from build123d import *

# Parameters (mm, degrees)
SKETCH1_R           = 5.5
BOSS_EXTRUDE1_DEPTH = 14
SKETCH2_R           = 5.5
BOSS_EXTRUDE2_DEPTH = 13.52
SKETCH3_R           = 5.5
BOSS_EXTRUDE3_DEPTH = 5.8
SKETCH4_R           = 1.05
CUT_EXTRUDE1_DEPTH  = 3.5


with BuildPart() as part:
    # Sketch1 → Boss-Extrude1 (new body)
    with BuildSketch(Plane.YZ):
        with Locations(Location((0, 0, 0), (0, 0, 270))):
            Circle(SKETCH1_R)
        with BuildLine():
            Line((-1.747140521, 2.5), (1.747140521, 2.5))
            ThreePointArc((1.747140521, 2.5), (0, -3.05), (-1.747140521, 2.5))
        make_face(mode=Mode.SUBTRACT)
    extrude(amount=BOSS_EXTRUDE1_DEPTH)

    # Sketch2 → Boss-Extrude2 (add)
    with BuildSketch(Plane.YZ.offset(14)):
        with Locations(Location((0, 0, 0), (0, 0, 270))):
            Circle(SKETCH2_R)
    extrude(amount=BOSS_EXTRUDE2_DEPTH)

    # Sketch3 → Boss-Extrude3 (add)
    with BuildSketch(Plane.YZ.offset(27.52)):
        with Locations(Location((0, 0, 0), (0, 0, 270))):
            Circle(SKETCH3_R)
        with BuildLine():
            ThreePointArc((-1.322019746, -2.893008891), (-1.318956528, -2.868853063), (-1.317084788, -2.844575833))
            ThreePointArc((-1.317084788, -2.844575833), (-1.543809469, -2.402214423), (-2.040380396, -2.37974197))
            ThreePointArc((-2.040380396, -2.37974197), (-2.061686193, -2.391529691), (-2.0823866, -2.404350785))
            ThreePointArc((-2.0823866, -2.404350785), (-2.380259348, -2.555545236), (-2.703854763, -2.638454478))
            ThreePointArc((-2.703854763, -2.638454478), (-2.855120731, -2.473976197), (-2.996397469, -2.300842198))
            ThreePointArc((-2.996397469, -2.300842198), (-2.868279694, -1.992339732), (-2.676232473, -1.719016114))
            ThreePointArc((-2.676232473, -1.719016114), (-2.660595904, -1.700351039), (-2.645896034, -1.680939672))
            ThreePointArc((-2.645896034, -1.680939672), (-2.597470339, -1.186224957), (-3.003062861, -0.898853414))
            ThreePointArc((-3.003062861, -0.898853414), (-3.02735936, -0.897251093), (-3.051705258, -0.896845399))
            ThreePointArc((-3.051705258, -0.896845399), (-3.384033651, -0.862996099), (-3.701083558, -0.757794901))
            ThreePointArc((-3.701083558, -0.757794901), (-3.739412915, -0.537646409), (-3.764659163, -0.315616851))
            ThreePointArc((-3.764659163, -0.315616851), (-3.490090608, -0.12535376), (-3.1807603, 0.000752133))
            ThreePointArc((-3.1807603, 0.000752133), (-3.157514879, 0.008000426), (-3.134653985, 0.016382957))
            ThreePointArc((-3.134653985, 0.016382957), (-2.82645273, 0.406382552), (-3.012294086, 0.86741475))
            ThreePointArc((-3.012294086, 0.86741475), (-3.031867321, 0.881898388), (-3.052129059, 0.895402065))
            ThreePointArc((-3.052129059, 0.895402065), (-3.31340118, 1.103548202), (-3.523244473, 1.363459202))
            ThreePointArc((-3.523244473, 1.363459202), (-3.43646792, 1.569382314), (-3.337668173, 1.769814617))
            ThreePointArc((-3.337668173, 1.769814617), (-3.003822413, 1.781431146), (-2.675419206, 1.720281583))
            ThreePointArc((-2.675419206, 1.720281583), (-2.65194519, 1.713811812), (-2.628181444, 1.708504114))
            ThreePointArc((-2.628181444, 1.708504114), (-2.158056349, 1.869966471), (-2.065143222, 2.35828486))
            ThreePointArc((-2.065143222, 2.35828486), (-2.07377883, 2.381051361), (-2.083523449, 2.4033657))
            ThreePointArc((-2.083523449, 2.4033657), (-2.190787246, 2.719723746), (-2.226800162, 3.051824643))
            ThreePointArc((-2.226800162, 3.051824643), (-2.042468641, 3.178143241), (-1.850991121, 3.293342448))
            ThreePointArc((-1.850991121, 3.293342448), (-1.563861826, 3.12262425), (-1.320651417, 2.893633786))
            ThreePointArc((-1.320651417, 2.893633786), (-1.304401641, 2.875500057), (-1.287279864, 2.858187286))
            ThreePointArc((-1.287279864, 2.858187286), (-0.804492326, 2.739849249), (-0.462323977, 3.100416189))
            ThreePointArc((-0.462323977, 3.100416189), (-0.457280213, 3.124237351), (-0.453413865, 3.148277707))
            ThreePointArc((-0.453413865, 3.148277707), (-0.372613841, 3.472406218), (-0.223362534, 3.771257322))
            ThreePointArc((-0.223362534, 3.771257322), (-0.111730141, 3.776213578), (0, 3.777866145))
            ThreePointArc((0, 3.777866145), (0.111730141, 3.776213578), (0.223362534, 3.771257322))
            ThreePointArc((0.223362534, 3.771257322), (0.372613841, 3.472406218), (0.453413865, 3.148277707))
            ThreePointArc((0.453413865, 3.148277707), (0.457280213, 3.124237351), (0.462323977, 3.100416189))
            ThreePointArc((0.462323977, 3.100416189), (0.804492326, 2.739849249), (1.287279864, 2.858187286))
            ThreePointArc((1.287279864, 2.858187286), (1.304401641, 2.875500057), (1.320651417, 2.893633786))
            ThreePointArc((1.320651417, 2.893633786), (1.563861826, 3.12262425), (1.850991121, 3.293342448))
            ThreePointArc((1.850991121, 3.293342448), (2.042468641, 3.178143241), (2.226800162, 3.051824643))
            ThreePointArc((2.226800162, 3.051824643), (2.190787246, 2.719723746), (2.083523449, 2.4033657))
            ThreePointArc((2.083523449, 2.4033657), (2.07377883, 2.381051361), (2.065143222, 2.35828486))
            ThreePointArc((2.065143222, 2.35828486), (2.158056349, 1.869966471), (2.628181444, 1.708504114))
            ThreePointArc((2.628181444, 1.708504114), (2.65194519, 1.713811812), (2.675419206, 1.720281583))
            ThreePointArc((2.675419206, 1.720281583), (3.003822413, 1.781431146), (3.337668173, 1.769814617))
            ThreePointArc((3.337668173, 1.769814617), (3.43646792, 1.569382314), (3.523244473, 1.363459202))
            ThreePointArc((3.523244473, 1.363459202), (3.31340118, 1.103548202), (3.052129059, 0.895402065))
            ThreePointArc((3.052129059, 0.895402065), (3.031867321, 0.881898388), (3.012294086, 0.86741475))
            ThreePointArc((3.012294086, 0.86741475), (2.82645273, 0.406382552), (3.134653985, 0.016382957))
            ThreePointArc((3.134653985, 0.016382957), (3.157514879, 0.008000426), (3.1807603, 0.000752133))
            ThreePointArc((3.1807603, 0.000752133), (3.490090608, -0.12535376), (3.764659163, -0.315616851))
            ThreePointArc((3.764659163, -0.315616851), (3.739412915, -0.537646409), (3.701083558, -0.757794901))
            ThreePointArc((3.701083558, -0.757794901), (3.384033651, -0.862996099), (3.051705258, -0.896845399))
            ThreePointArc((3.051705258, -0.896845399), (3.02735936, -0.897251093), (3.003062861, -0.898853414))
            ThreePointArc((3.003062861, -0.898853414), (2.597470339, -1.186224957), (2.645896034, -1.680939672))
            ThreePointArc((2.645896034, -1.680939672), (2.660595904, -1.700351039), (2.676232473, -1.719016114))
            ThreePointArc((2.676232473, -1.719016114), (2.868279694, -1.992339732), (2.996397469, -2.300842198))
            ThreePointArc((2.996397469, -2.300842198), (2.855120731, -2.473976197), (2.703854763, -2.638454478))
            ThreePointArc((2.703854763, -2.638454478), (2.380259349, -2.555545235), (2.082386604, -2.404350784))
            ThreePointArc((2.082386604, -2.404350784), (2.061686196, -2.39152969), (2.0403804, -2.379741969))
            ThreePointArc((2.0403804, -2.379741969), (1.54380947, -2.402214422), (1.317084788, -2.844575834))
            ThreePointArc((1.317084788, -2.844575834), (1.318956528, -2.868853064), (1.322019746, -2.893008892))
            ThreePointArc((1.322019746, -2.893008892), (1.335810244, -3.226771918), (1.27680075, -3.555566405))
            ThreePointArc((1.27680075, -3.555566405), (1.064347889, -3.624836022), (0.848171186, -3.6814234))
            ThreePointArc((0.848171186, -3.6814234), (0.62076952, -3.436726817), (0.45192491, -3.148491786))
            ThreePointArc((0.45192491, -3.148491786), (0.441442226, -3.12651451), (0.429891573, -3.105079266))
            ThreePointArc((0.429891573, -3.105079266), (0, -2.855517783), (-0.429891573, -3.105079265))
            ThreePointArc((-0.429891573, -3.105079265), (-0.441442226, -3.12651451), (-0.45192491, -3.148491786))
            ThreePointArc((-0.45192491, -3.148491786), (-0.62076952, -3.436726817), (-0.848171186, -3.6814234))
            ThreePointArc((-0.848171186, -3.6814234), (-1.064347889, -3.624836022), (-1.27680075, -3.555566405))
            ThreePointArc((-1.27680075, -3.555566405), (-1.335810244, -3.226771917), (-1.322019746, -2.893008891))
        make_face(mode=Mode.SUBTRACT)
    extrude(amount=BOSS_EXTRUDE3_DEPTH)

    # Sketch4 → Cut-Extrude1 (cut)
    with BuildSketch(Plane.YZ.offset(27.52)):
        with Locations(Location((0, 0, 0), (0, 0, 270))):
            Circle(SKETCH4_R)
    extrude(amount=-CUT_EXTRUDE1_DEPTH, mode=Mode.SUBTRACT)


solid = part.part
Here's how the part is built. I have some questions about the finished solid (model axes, mm). A direction names the side the tool comes from. Round coordinates to 2 decimals unless told otherwise and drop trailing zeros. Loops run counter-clockwise (first coordinate to the right, second up) from the corner with the lowest first, then second, coordinate; pieces in that order, holes last.
1. For P1, Ø4.5, axis at y = 1, z = 0.5, coming from the -X side; P2, Ø2, axis at x = 13.5, y = 4, coming from the -Z side; P3, Ø6, axis at x = 8.5, y = -3.5, coming from the +Z side; P4, Ø2.5, axis at y = 0, z = 0, coming from the +X side, each with a flat end and sliding along its axis, tell me the tip position at first contact or that it passes through.
Answer list:
P1: stops at x = 0
P2: stops at z = -4.61
P3: stops at z = 5.48
P4: stops at x = 27.52
2. If we section it at C-C on x = 13.5: Write out the boundary of the cut face in (y, z), plus the area to 3 significant figures.
Answer list:
outline: circle Ø11 at (0, 0); hole (-1.75, 2.5) arc R3.05 ccw (long way) to (1.75, 2.5) - close
area: 67.1 mm2
3. Which directions (+Z, -Z, +X, -X, +Y, -Y) give clear straight access to the entire face, cutting with the end or side of a thin tool? Please do faces 1 (the face through (24.02, 0, 0)), 2 (the face through (0, 0, 3)), 3 (the face through (14, 0, 0)).
Answer list:
face 1: +X
face 2: +Z, -Z, -X, +Y, -Y
face 3: -X
4. If we section it at D-D on z = -4.5: Write out the boundary of the cut face in (x, y).
Answer list:
outline: (0, -3.16) - (33.32, -3.16) - (33.32, 3.16) - (0, 3.16) - close
5. If we section it at B-B on z = 4.75: Write out the boundary of the cut face in (x, y), plus the area to 3 significant figures.
Answer list:
outline: (0, -2.77) - (33.32, -2.77) - (33.32, 2.77) - (0, 2.77) - close
area: 185 mm2
6. If I drill on line 1 along Y through (x, z) = (8.5, 0); line 2 along Y through (x, z) = (26.1, 0); line 3 along Z through (x, y) = (8, 2.5), over which ranges is the centre line in solid material (lowest first)?
Answer list:
line 1: y = -5.5 to -3.05, 3.05 to 5.5
line 2: y = -5.5 to -1.05, 1.05 to 5.5
line 3: z = -4.9 to -1.75, 1.75 to 4.9
7. We'd pull the mould along Z, two halves only. Please class faces 4 (the face through (33.32, -2.4, 2.5)), 5 (the face through (16.43, -5.37, 1.19)), 6 (the face through (6.9, 0.11, -3.05)): +Z half, -Z half, draft (parallel to the pull), parting line (faces both ways), or undercut.
Answer list:
face 4: draft
face 5: parting line
face 6: undercut
8. If we section it at A-A on x = 25.5: Write out the boundary of the cut face in (y, z).
Answer list:
outline: circle Ø11 at (0, 0); hole circle Ø2.1 at (0, 0)
